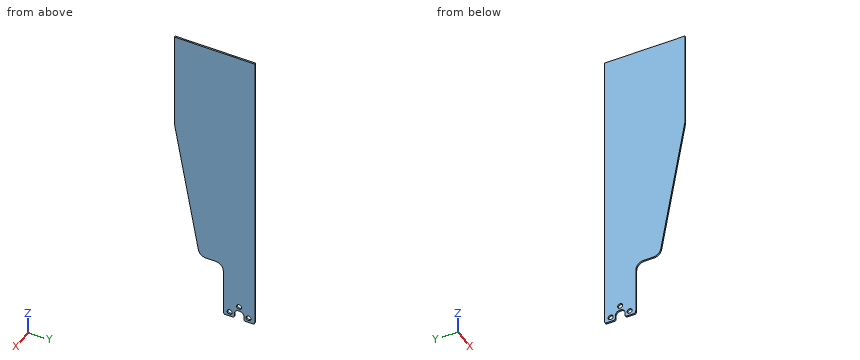
Autodesk Inventor part; units mm, degrees
ref_plane "YZ Plane" through (0, 0, 0) normal (1, 0, 0) x (0, 1, 0)
ref_plane "XZ Plane" through (0, 0, 0) normal (0, 1, 0) x (-1, 0, 0)
ref_plane "XY Plane" through (0, 0, 0) normal (0, 0, 1) x (1, 0, 0)
sketch "スケッチ1" plane through (0, 0, 0) normal (1, 0, 0) x (0, 1, 0)
  line L0 (-41, 550) -> (10, 550)
  line L1 (10, 550) -> (10, -10)
  line L2 (10, -10) -> (-41, -10)
  line L3 (-41, -10) -> (-41, 550)
  line L4 (-41, 550) -> (10, -10) construction
  line L5 (10, 550) -> (-41, -10) construction
  point P0 (0, 0)
  dimension "d0" = 51
  dimension "d1" = 560
  dimension "d42" = 10
  dimension "d43" = 10
extrude "プレート1" add sketch "スケッチ1" along normal mid plane 1
sketch "スケッチ3" plane through (0.5, 0, 0) normal (1, 0, 0) x (0, 0, -1)
  circle A0 centre (0, 0) radius 6
  line L0 (10, 10) -> (10, -41)
  line L1 (-550, 10) -> (10, 10)
  point P0 (0, 0)
  point P1 (0, 6)
  point P2 (-6, 0)
  point P3 (0, -6)
  point P4 (6, 0)
  dimension "d13" = 12
  dimension "d14" = 10
  dimension "d15" = 10
  dimension "d18" = 360
  dimension "d44" = 0
hole "穴2" at (0.5, 6, 0) at (0.5, 0, 6) at (0.5, -6, 0) at (0.5, 0, -6) direction (-1, 0, 0) diameter 3.2 end through all
sketch "スケッチ4" plane through (0.5, 0, 0) normal (1, 0, 0) x (0, 0, -1)
  circle A0 centre (0, 0) radius 3.05
  point P0 (0, 0)
  dimension "d27" = 6.1
extrude "押し出し1" cut sketch "スケッチ4" against normal blind 10
sketch "スケッチ5" plane through (0.5, 0, 0) normal (1, 0, 0) x (0, 0, -1)
  line L0 (10, -41) -> (-33.5, -41)
  line L1 (-33.5, -41) -> (-33.5, -10)
  line L2 (-33.5, -10) -> (10, -10)
  line L3 (10, -10) -> (10, -41)
  line L4 (-550, 10) -> (-53.5, 10)
  line L5 (-53.5, 10) -> (-53.5, -12)
  line L6 (-53.5, -12) -> (-550, -12)
  line L7 (-550, -12) -> (-550, 10)
  line L8 (10, -41) -> (-550, -41)
  circle A0 centre (0, 0) radius 3.05
  circle A1 centre (0, 0) radius 3.05
  line L9 (0, 3.05) -> (10, 3.05)
  line L10 (0, -3.05) -> (10, -3.05)
  line L11 (10, 10) -> (10, -41)
  circle A2 centre (0, 0) radius 10
  circle A3 centre (0, 6) radius 1.6
  circle A4 centre (0, -6) radius 1.6
  line L12 (-550, 10) -> (10, 10)
  line L13 (2.95, 10) -> (2.95, -10)
  point P0 (0, 0)
  point P1 (2.95, -3.05)
  point P2 (2.95, 3.05)
  point P3 (2.95, 0.7746)
  point P4 (2.95, -0.7746)
  point P5 (9.5235, -3.05)
  point P6 (0, -10)
  point P7 (0, 10)
  point P8 (9.5235, 3.05)
  point P9 (10, 0)
  point P10 (2.95, -9.555)
  point P11 (2.95, 9.555)
  dimension "d35" = 29
  dimension "d36" = 20
  dimension "d40" = 33.5
  dimension "d41" = 10
  dimension "d45" = 2.95
extrude "押し出し2" cut sketch "スケッチ5" against normal blind 10 contours L0 L1 L2 L3 | L2 L13 A2 L10 L11 | L2 A2 L13 | L10 A2 L11 | L13 L10 A2 | L10 L13 A0 L9 A2 | A2 L9 L11 | L12 L13 A2 | L10 A0 L13 | L9 A2 L13 L12 L11 | L9 L13 A2 | L13 A0 L9 picked at (5.1412, -2.2915)
fillet "コーナーR4" radius 1 4 edges at (0, -3.05, -2.95) (0, 3.05, -2.95) (0, 9.555, -2.95) (0, -9.555, -2.95)
sketch "スケッチ6" plane through (0.5, 0, 0) normal (1, 0, 0) x (0, 0, -1)
  line L0 (-33.5, -41) -> (-550, -41)
  line L1 (-33.5, -41) -> (-33.5, -10)
  line L2 (-33.5, -25) -> (-124.2405, -41)
  point P0 (0, 0)
  point P1 (-545, -41)
  point P2 (-33.5, -15)
  dimension "d51" = 10
  dimension "d52" = 16
extrude "押し出し3" cut sketch "スケッチ6" against normal blind 10
fillet "コーナーR5" radius 5 2 edges at (0, -25, 33.5) (0, -41, 124.2405)
fillet "コーナーR6" radius 5 2 edges at (0, -10, 33.5) (0, 10, 550)
ref_plane "作業平面1" through (0.5, 4.05, 187.05) normal (0, 0, -1) x (-1, 0, 0)
sketch "スケッチ7" plane through (0.5, 4.05, 187.05) normal (0, 0, -1) x (-1, 0, 0)
  line L0 (1, -45.05) -> (0, -45.05)
  line L1 (0, -45.05) -> (1, -45.05)
  line L2 (1, -45.05) -> (1, 5.95)
  line L3 (1, 5.95) -> (0, 5.95)
  line L4 (0, 5.95) -> (0, -45.05)
  point P0 (0.5, -4.05)
  point P1 (1, -45.05)
extrude "押し出し4" cut sketch "スケッチ7" against normal through all
equation "\"d25\" = Thickness"
equation "\"d2\" = Thickness"
equation "\"BendRadius\" = Thickness"
equation "\"BendReliefWidth\" = Thickness"
equation "\"BendReliefDepth\" = 0.5 * Thickness"
equation "\"CornerReliefSize\" = 4 * Thickness"
equation "\"MinimumRemnant\" = 2 * Thickness"
equation "\"TransitionRadius\" = BendRadius"
equation "\"JacobiRadiusSize\" = BendRadius"
equation "\"GapSize\" = Thickness"
properties part number "s_carbon_plate5" material "CFRP"
The model under review builds one solid part; all positions refer to its coordinate system, in mm. Round coordinates to 2 decimals unless told otherwise and drop trailing zeros. Order: outer loops, then holes, each group sorted by start corner. A loop starts at its lowest first (then second) coordinate and runs counter-clockwise, first axis right, second up. Notation, with made-up numbers: (80.25, -12.75) -> (94.25, -12.75) arc R20 ccw to (94.25, 25.25) -> close; hole circle Ø3 at (-19, -32.5). An arc over 180 degrees is marked (long way). Use a Markdown table: item, result.
Q1. We need section C-C on x = -0.05. Write out the cut boundary in (y, z), then the cut area to 3 significant figures.
Values:
| item | result |
|---|---|
| outline | (-41, 124.68) arc R5 ccw to (-40.92, 123.81) -> (-25.73, 37.63) arc R5 ccw to (-20.8, 33.5) -> (-15, 33.5) arc R5 cw to (-10, 28.5) -> (-10, 0) arc R10 ccw to (-9.76, -2.17) arc R1 ccw to (-8.79, -2.95) -> (-4.05, -2.95) arc R1 ccw to (-3.05, -1.95) -> (-3.05, 0) arc R3.05 cw to (3.05, 0) -> (3.05, -1.95) arc R1 ccw to (4.05, -2.95) -> (8.79, -2.95) arc R1 ccw to (9.76, -2.17) arc R10 ccw to (10, 0) -> (10, 187.05) -> (-41, 187.05) -> close; hole circle Ø3.2 at (-6, 0); hole circle Ø3.2 at (0, 6); hole circle Ø3.2 at (6, 0) |
| area | 7,780 mm^2 |
Q2. We need section D-D on y = -31.5. Write out the cut boundary in (x, z), then the cut area to 3 significant figures.
Values:
| item | result |
|---|---|
| outline | (-0.5, 70.36) -> (0.5, 70.36) -> (0.5, 187.05) -> (-0.5, 187.05) -> close |
| area | 117 mm^2 |
Q3. For line 1 (Y direction, x = -0.1, z = 0); line 2 (Z direction, x = -0.05, y = -6); line 3 (Y direction, x = 0.05, z = 6), list the stretches that pass through material, from the lowest coordinate up.
Values:
| item | result |
|---|---|
| line 1 | y = -10 to -7.6, -4.4 to -3.05, 3.05 to 4.4, 7.6 to 10 |
| line 2 | z = -2.95 to -1.6, 1.6 to 187.05 |
| line 3 | y = -10 to -1.6, 1.6 to 10 |
Q4. We need section A-A on z = 6. Write out the cut boundary in (x, y).
Values:
| item | result |
|---|---|
| outline | (-0.5, -10) -> (0.5, -10) -> (0.5, -1.6) -> (-0.5, -1.6) -> close; (-0.5, 1.6) -> (0.5, 1.6) -> (0.5, 10) -> (-0.5, 10) -> close |
Q5. We need section B-B on y = -6. Write out the cut boundary in (x, z).
Values:
| item | result |
|---|---|
| outline | (-0.5, -2.95) -> (0.5, -2.95) -> (0.5, -1.6) -> (-0.5, -1.6) -> close; (-0.5, 1.6) -> (0.5, 1.6) -> (0.5, 187.05) -> (-0.5, 187.05) -> close |
Q6. Clearance check with flat-ended pins moving along their axes: P1, Ø6, axis at y = -27, z = 35, coming from the +X side; P2, Ø0.5, axis at x = 0, z = -0.5, coming from the -Y side; P3, Ø0.5, axis at x = 0, y = -19, coming from the -Z side. State where each tip first meets the part, or that it passes through.
Values:
| item | result |
|---|---|
| P1 | stops at x = 0.5 |
| P2 | stops at y = -10 |
| P3 | stops at z = 33.5 |
